from build123d import *

# Parameters (mm, degrees)
ESQUISSE1_W             = 50
ESQUISSE1_H             = 284
BOSS_EXTRU_1_DEPTH      = 8
ESQUISSE2_R             = 3
ENL_V_MAT_EXTRU_1_DEPTH = 289.478768716
ESQUISSE3_W             = 2
ESQUISSE3_H             = 30
BOSS_EXTRU_2_DEPTH      = 8
CHANFREIN1_SIZE         = 2
ESQUISSE4_R             = 2.25
ENL_V_MAT_EXTRU_2_DEPTH = 289.832131177
ESQUISSE5_R             = 1.75
ENL_V_MAT_EXTRU_3_DEPTH = 289.832131177


with BuildPart() as part:
    # Esquisse1 → Boss.-Extru.1 (new body)
    with BuildSketch(Plane.XY):
        with Locations((25, 142)):
            Rectangle(ESQUISSE1_W, ESQUISSE1_H)
    extrude(amount=BOSS_EXTRU_1_DEPTH)

    # Esquisse2 → Enlèv. mat.-Extru.1 (cut, through all)
    with BuildSketch(Plane.XY.offset(8)):
        with Locations((3.5, 18)):
            Circle(ESQUISSE2_R)
        with Locations(Location((46.5, 18, 0), (0, 0, 180))):
            Circle(ESQUISSE2_R)
        with Locations((46.5, 266)):
            Circle(ESQUISSE2_R)
        with Locations(Location((3.5, 266, 0), (0, 0, 180))):
            Circle(ESQUISSE2_R)
    extrude(amount=-ENL_V_MAT_EXTRU_1_DEPTH, mode=Mode.SUBTRACT)

    # Esquisse3 → Boss.-Extru.2 (add)
    with BuildSketch(Plane.XY.offset(8)):
        with Locations((-1, 15)):
            Rectangle(ESQUISSE3_W, ESQUISSE3_H)
        with Locations((51, 15)):
            Rectangle(ESQUISSE3_W, ESQUISSE3_H)
        with Locations((51, 269)):
            Rectangle(ESQUISSE3_W, ESQUISSE3_H)
        with Locations((-1, 269)):
            Rectangle(ESQUISSE3_W, ESQUISSE3_H)
    extrude(amount=-BOSS_EXTRU_2_DEPTH)

    # Chanfrein1
    chanfrein1_edges = [part.edges().sort_by_distance(p)[0] for p in [
        (50, 30, 4),
        (0, 30, 4),
        (0, 254, 4),
        (50, 254, 4),
    ]]
    chamfer(chanfrein1_edges, length=CHANFREIN1_SIZE - 0.0001)  # a hair under: the kernel refuses the full size

    # Esquisse4 → Enlèv. mat.-Extru.2 (cut, through all)
    with BuildSketch(Plane.XY.offset(8)):
        with Locations((10, 41.5)):
            Circle(ESQUISSE4_R)
        with Locations((10, 88)):
            Circle(ESQUISSE4_R)
        with Locations(Location((40, 88, 0), (0, 0, 180))):
            Circle(ESQUISSE4_R)
        with Locations(Location((40, 41.5, 0), (0, 0, 180))):
            Circle(ESQUISSE4_R)
        with Locations((40, 242.5)):
            Circle(ESQUISSE4_R)
        with Locations((40, 196)):
            Circle(ESQUISSE4_R)
        with Locations(Location((10, 196, 0), (0, 0, 180))):
            Circle(ESQUISSE4_R)
        with Locations(Location((10, 242.5, 0), (0, 0, 180))):
            Circle(ESQUISSE4_R)
    extrude(amount=-ENL_V_MAT_EXTRU_2_DEPTH, mode=Mode.SUBTRACT)

    # Esquisse5 → Enlèv. mat.-Extru.3 (cut, through all)
    with BuildSketch(Plane.XY.offset(8)):
        with Locations((44.5, 215)):
            Circle(ESQUISSE5_R)
        with Locations((31, 215)):
            Circle(ESQUISSE5_R)
        with Locations(Location((17.5, 215, 0), (0, 0, 180))):
            Circle(ESQUISSE5_R)
    extrude(amount=-ENL_V_MAT_EXTRU_3_DEPTH, mode=Mode.SUBTRACT)


solid = part.part
Input: part model. Units: mm. Frame: model coordinates. A direction names the side the tool comes from. Give positions to 0.01 mm unless a question says otherwise; leave off trailing zeros. Write each loop counter-clockwise with the first axis right and the second up, starting at its lowest first coordinate (ties: lowest second). Pieces come first, ordered by that corner, then holes. Notation, with made-up numbers: M 83,80.5 L 109,80.5 A19 ccw 109,95.5 Z; hole C 89,49.25 d1. An arc over 180 degrees is marked long. Write item = value, one per line. Start each with the question number.
1) First-contact query: pin 1 Ø4 at (y, z) = (162, 5) entering from -X; pin 2 Ø4 at (y, z) = (187.5, 2.5) entering from +X. Flat tips, straight axial feed; report the tip coordinate or a pass-through.
2) Draft query along Y for faces 3 (the flat face through (25, 144, 0)), 4 (the cylindrical face through (39.71, 244.73, 4.06)), 5 (the flat face through (25, 284, 4)), 6 (the flat face through (50, 140, 4)). Return one class per face: +Y half, -Y half, draft (parallel to the pull), parting line (faces both ways), or undercut.
3) Reachability of faces 1 (the flat face through (0, 140, 4)), 2 (the cylindrical face through (2.85, 15.07, 4.06)) from +Z, -Z, +X, -X, +Y, -Y: full face, straight path, thin tool, end or side. Return the list, or none.
4) Cut plane C-C on z = 1.75. Count the separate pieces of the cut face and the enclosed holes in it, then the cut area to 3 significant figures.
5) Cut plane A-A on x = 3.5. Return the cut outline in (y, z).
6) Cut plane B-B on y = 266. Return the cut outline in (x, z), then the cut area to 3 significant figures.
7) Cut plane D-D on y = 101. Return the cut outline in (x, z).
8) Material intervals for line 1 along X through (y, z) = (215, 3.5); line 2 along Y through (x, z) = (46.5, 4.5); line 3 along Y through (x, z) = (44.5, 3.75), sorted ascending. Write a range as [from, to].
Solved:
q1.pin_1 = 0
q1.pin_2 = 50
q2.face_3 = draft
q2.face_4 = undercut
q2.face_5 = +Y half
q2.face_6 = undercut
q3.face_1 = +Z, -Z, -X
q3.face_2 = +Z, -Z
q4.separate_pieces = 1
q4.enclosed_holes = 15
q4.area = 14,200 mm2
q5.outline = M 0,0 L 15,0 L 15,8 L 0,8 Z; M 21,0 L 263,0 L 263,8 L 21,8 Z; M 269,0 L 284,0 L 284,8 L 269,8 Z
q6.outline = M -2,0 L 0.5,0 L 0.5,8 L -2,8 Z; M 6.5,0 L 43.5,0 L 43.5,8 L 6.5,8 Z; M 49.5,0 L 52,0 L 52,8 L 49.5,8 Z
q6.area = 336 mm2
q7.outline = M 0,0 L 50,0 L 50,8 L 0,8 Z
q8.line_1 = [0, 15.75], [19.25, 29.25], [32.75, 42.75], [46.25, 50]
q8.line_2 = [0, 15], [21, 263], [269, 284]
q8.line_3 = [0, 15.76], [20.24, 213.25], [216.75, 263.76], [268.24, 284]
